from build123d import *

# Parameters (mm, degrees)
F2_W     = 30
F2_H     = 30
F2_R     = 1.55
F2_R_2   = 12
F3_DEPTH = 2.5
F4_R     = 3


with BuildPart() as f1:
    # F0 (on Right) → F1 (revolve)
    with BuildSketch(Plane.YZ):
        with BuildLine():
            ThreePointArc((0, 12), (-8.4852813742, 8.4852813742), (-12, 0))
            Line((-12, 0), (0, 0))
            Line((0, 0), (0, 12))
        make_face()
    revolve(axis=Axis((0, 0, 6), (0, 0, 1)))

    # F2 (on face) → F3 (join)
    with BuildSketch(Plane(origin=(0, 0, 0), x_dir=(1, 0, 0), z_dir=(0, 0, -1))):
        Rectangle(F2_W, F2_H)
        with Locations((-10.6066017178, -10.6066017178)):
            Circle(F2_R, mode=Mode.SUBTRACT)
        with Locations((10.6066017178, -10.6066017178)):
            Circle(F2_R, mode=Mode.SUBTRACT)
        with Locations((-10.6066017178, 10.6066017178)):
            Circle(F2_R, mode=Mode.SUBTRACT)
        Circle(F2_R_2, mode=Mode.SUBTRACT)
        with Locations((10.6066017178, 10.6066017178)):
            Circle(F2_R, mode=Mode.SUBTRACT)
        Circle(F2_R_2)
    extrude(amount=F3_DEPTH)

    # F4
    f4_edges = [f1.edges().sort_by_distance(p)[0] for p in [
        (15, 15, -1.25),
        (-15, 15, -1.25),
        (15, -15, -1.25),
        (-15, -15, -1.25),
    ]]
    fillet(f4_edges, radius=F4_R)


solid = f1.part
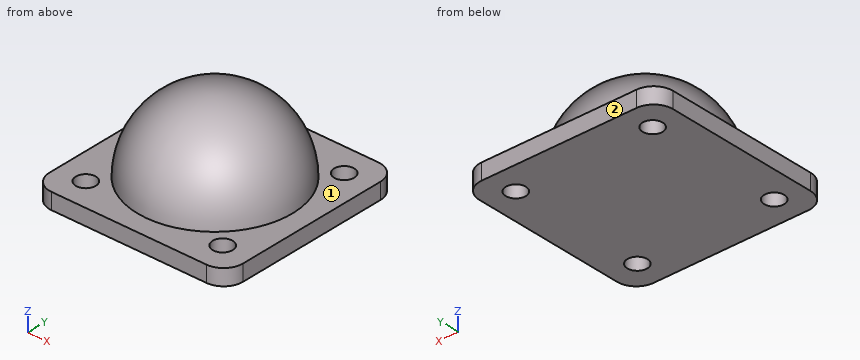
For this review, take the finished solid that the model builds, in its own axes (mm). Face numbers are marked on the shaded views. A direction names the side the tool comes from. Round coordinates to 2 decimals unless told otherwise and drop trailing zeros. Loops run counter-clockwise (first coordinate to the right, second up) from the corner with the lowest first, then second, coordinate; pieces in that order, holes last. Notation, with made-up numbers: (3, -22.5) - (51, -22.5) arc R25 ccw to (51, -7.5) - close; hole circle Ø4 at (80.5, 6.5). An arc over 180 degrees is marked (long way). One line per item, written item: value. Start each with the question number.
Item 1: Take a section at A-A (x = 10.25). Give the boundary of the cut face in (y, z), plus the area to 3 significant figures.
Item 2: Take a section at C-C (x = 6). Give the boundary of the cut face in (y, z), plus the area to 3 significant figures.
Item 3: Take a section at B-B (y = 5.5). Give the boundary of the cut face in (x, z).
Item 4: For the marked faces 1 and 2, list the 3-axis set-ups (+Z, -Z, +X, -X, +Y, -Y) from which the entire face can be reached by the end or side of a thin tool; tool diameter is ignored.
Item 5: For L1, parallel to Z at x = 8.25, y = 10; L2, parallel to X at y = -8.25, z = 4; L3, parallel to Z at x = 5.75, y = -4, list the stretches that pass through material, from the lowest coordinate up.
Item 6: Clearance check with flat-ended pins moving along their axes: pin 1 Ø5 at (x, z) = (8.5, 2) entering from +Y; pin 2 Ø10 at (x, y) = (9.5, 11.5) entering from +Z; pin 3 Ø3.5 at (x, y) = (10.61, -10.61) entering from +Z; pin 4 Ø5 at (x, z) = (-6.5, 4.5) entering from -Y. State where each tip first meets the part, or that it passes through.
Item 7: Take a section at D-D (z = 8.5). Give the boundary of the cut face in (x, y).
Answer below:
1. outline: (-15, -2.5) - (-12.12, -2.5) - (-12.12, 0) - (-15, 0) - close; (-9.1, -2.5) - (9.1, -2.5) - (9.1, 0) - (6.24, 0) arc R6.24 ccw to (-6.24, 0) - (-9.1, 0) - close; (12.12, -2.5) - (15, -2.5) - (15, 0) - (12.12, 0) - close
1. area: 121 mm2
2. outline: (-15, -2.5) - (15, -2.5) - (15, 0) - (10.39, 0) arc R10.39 ccw to (-10.39, 0) - (-15, 0) - close
2. area: 245 mm2
3. outline: (-15, -2.5) - (15, -2.5) - (15, 0) - (10.67, 0) arc R10.67 ccw to (-10.67, 0) - (-15, 0) - close
4. face 1: +Z
4. face 2: +Z, -Z, +X, -X, +Y
5. L1: z = -2.5 to 0
5. L2: x = -7.74 to 7.74
5. L3: z = -2.5 to 9.74
6. pin 1: stops at y = 15
6. pin 2: stops at z = 6.76
6. pin 3: stops at z = 0
6. pin 4: stops at y = -10.71
7. outline: circle Ø16.94 at (0, 0)
